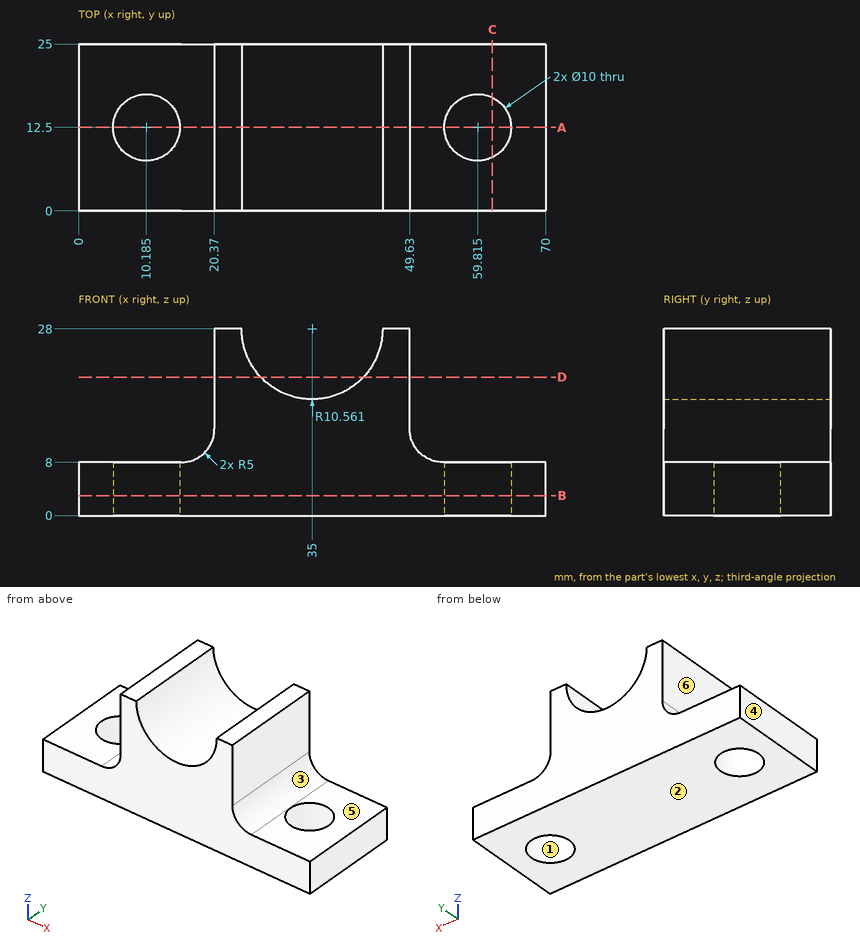
Check sheet for the drawn part. Datum: minimum x, y, z corner. Units: mm. A direction names the side the tool comes from. Give positions to 0.01 mm unless a question says otherwise; leave off trailing zeros. Order: outer loops, then holes, each group sorted by start corner. A loop starts at its lowest first (then second) coordinate and runs counter-clockwise, first axis right, second up. Notation, with made-up numbers: (1, -33.5) - (45, -33.5) arc R32 ccw to (45, -0.5) - close; hole circle Ø5 at (60.5, 75.25). An arc over 180 degrees is marked (long way). Answer in a Markdown table with one row per item. Add a question column.
Q1. Tool access check on the marked faces 4, 5 and 6. Record the directions out of +Z, -Z, +X, -X, +Y, -Y that give a thin tool (end or side, any length) a straight path to the whole face; none if there is none.
Q2. Cross-section at D-D, the plane z = 20.75. Enter the section's corners in (x, y).
Q3. Material ranges on probe 1 along X at (y, z) = (8.5, 4) (1 decimal); probe 2 along Z at (x, y) = (4.5, 12.5); probe 3 along X at (y, z) = (13.25, 6), recorded low to high. Write a range as from..to.
Q4. Cross-section at B-B, the plane z = 3. Enter the section's corners in (x, y) (1 decimal), then the cut area to 3 significant figures.
Q5. Cross-section at A-A, the plane y = 12.5. Count the separate pieces of the cut face and the enclosed holes in it, then the cut area to 3 significant figures.
Q6. Cross-section at C-C, the plane x = 62. Enter the section's corners in (y, z), then the cut area to 3 significant figures.
Q7. Gauge pin test, flat ends, axial feed: pin 1 (1 mm diameter, centred on y = 17, z = 14, fed in from -X); pin 2 (7.5 mm diameter, centred on x = 60.5, y = 8, fed in from +Z); pin 3 (12 mm diameter, centred on y = 6, z = 20, fed in from +X). Record the tip position at first contact, or that the pin passes through.
Q8. Mould release check, pull along X, two halves, no side actions. Record for the marked faces 1, 2 and 3: pulls with the +X half, pulls with the -X half, needs draft (parallel to the pull), parting line crosses it, or undercut.
Check values:
| question | item | result |
|---|---|---|
| 1 | face 4 | +Z, -Z, -X, +Y, -Y |
| 1 | face 5 | +Z, +X, +Y, -Y |
| 1 | face 6 | +Z, -X, +Y, -Y |
| 2 | outline | (20.37, 0) - (27.32, 0) - (27.32, 25) - (20.37, 25) - close; (42.68, 0) - (49.63, 0) - (49.63, 25) - (42.68, 25) - close |
| 3 | probe 1 | x = 0..7.2, 13.2..56.8, 62.8..70 |
| 3 | probe 2 | z = 0..8 |
| 3 | probe 3 | x = 0..5.24, 15.13..54.87, 64.76..70 |
| 4 | outline | (0, 0) - (70, 0) - (70, 25) - (0, 25) - close; hole circle Ø10 at (10.2, 12.5); hole circle Ø10 at (59.8, 12.5) |
| 4 | area | 1,590 mm^2 |
| 5 | separate pieces | 3 |
| 5 | enclosed holes | 0 |
| 5 | area | 821 mm^2 |
| 6 | outline | (0, 0) - (8, 0) - (8, 8) - (0, 8) - close; (17, 0) - (25, 0) - (25, 8) - (17, 8) - close |
| 6 | area | 128 mm^2 |
| 7 | pin 1 | stops at x = 20.37 |
| 7 | pin 2 | stops at z = 8 |
| 7 | pin 3 | stops at x = 49.63 |
| 8 | face 1 | undercut |
| 8 | face 2 | needs draft |
| 8 | face 3 | pulls with the +X half |
